The drawing under review shows one solid part. Ordinate dimensions are in mm from its lowest x, y, z. A direction names the side the tool comes from. Round coordinates to 2 decimals unless told otherwise and drop trailing zeros. Write each loop counter-clockwise with the first axis right and the second up, starting at its lowest first coordinate (ties: lowest second). Pieces come first, ordered by that corner, then holes. Notation, with made-up numbers: (30.5, 15.5) -> (55.5, 15.5) arc R13 ccw to (55.5, 28.5) -> close; hole circle Ø6 at (2, -3). An arc over 180 degrees is marked (long way). Answer in a Markdown table with one row per item.
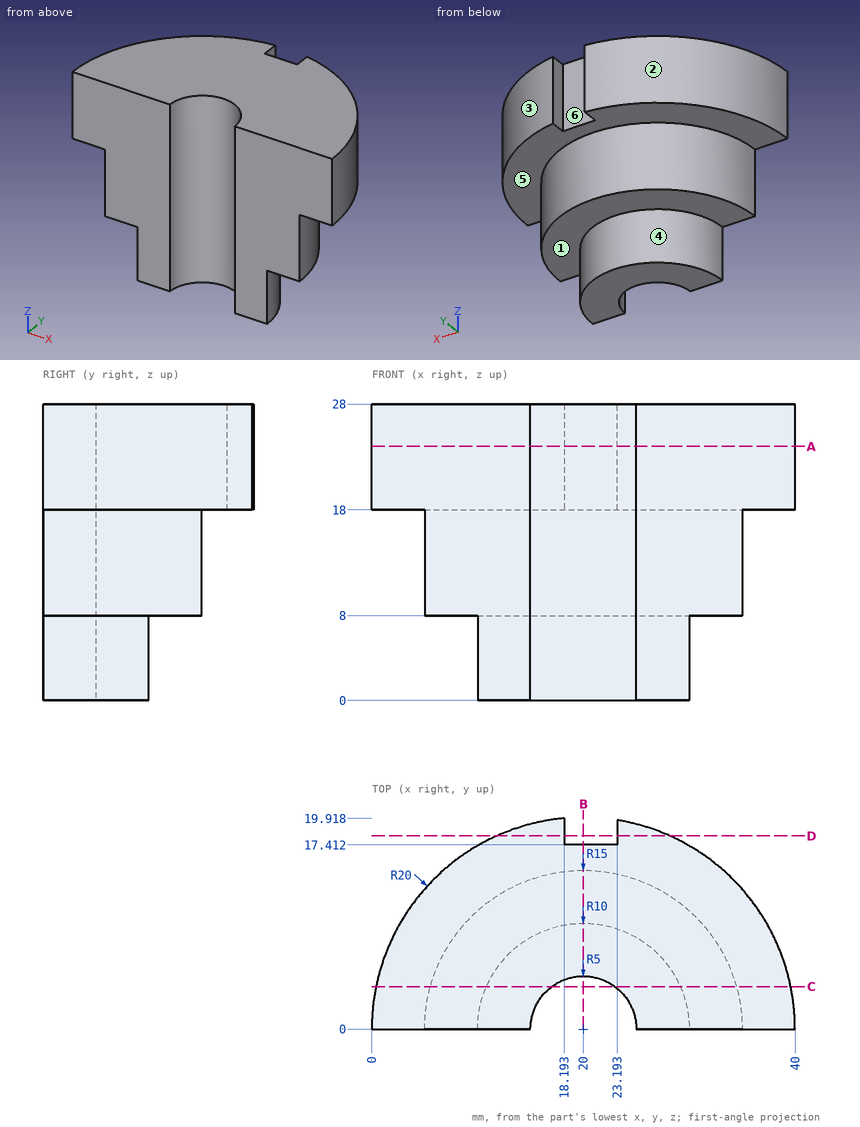
1) Mouldability with a two-part tool opening along X and no side actions: class the marked faces 3, 4, 5 and 6 as pulls with the +X half, pulls with the -X half, needs draft (parallel to the pull), parting line crosses it, or undercut.
Solved:
| item | result |
|---|---|
| face 3 | pulls with the +X half |
| face 4 | parting line crosses it |
| face 5 | needs draft |
| face 6 | undercut |
2) Consider section C-C on y = 4. State the section outline as (x, z) points (1 decimal).
Solved:
| item | result |
|---|---|
| outline | (0.4, 18) -> (5.5, 18) -> (5.5, 8) -> (10.8, 8) -> (10.8, 0) -> (17, 0) -> (17, 28) -> (0.4, 28) -> close; (23, 0) -> (29.2, 0) -> (29.2, 8) -> (34.5, 8) -> (34.5, 18) -> (39.6, 18) -> (39.6, 28) -> (23, 28) -> close |
3) Consider section D-D on y = 18.25. State the section outline as (x, z) points, then the cut area to 3 significant figures.
Solved:
| item | result |
|---|---|
| outline | (11.82, 18) -> (18.19, 18) -> (18.19, 28) -> (11.82, 28) -> close; (23.19, 18) -> (28.18, 18) -> (28.18, 28) -> (23.19, 28) -> close |
| area | 114 mm² |
4) For the marked faces 1 and 2, list the 3-axis set-ups (+Z, -Z, +X, -X, +Y, -Y) from which the entire face can be reached by the end or side of a thin tool; tool diameter is ignored.
Solved:
| item | result |
|---|---|
| face 1 | -Z, +Y |
| face 2 | +Z, -Z, -X, +Y |
5) Clearance check with flat-ended pins moving along their axes: pin 1 Ø2.5 at (x, z) = (20.5, 24.5) entering from +Y; pin 2 Ø1.5 at (x, y) = (13, 13.5) entering from -Z; pin 3 Ø2 at (y, z) = (4, 16.5) entering from -X. State where each tip first meets the part, or that it passes through.
Solved:
| item | result |
|---|---|
| pin 1 | y = 17.41 |
| pin 2 | z = 8 |
| pin 3 | x = 5.3 |
6) For line 1 (Z direction, x = 6.5, y = 13.25); line 2 (Z direction, x = 29, y = 7); line 3 (X direction, y = 1, z = 14.5), list the stretches that pass through material, from the lowest coordinate up. Write a range as [from, to].
Solved:
| item | result |
|---|---|
| line 1 | [18, 28] |
| line 2 | [8, 28] |
| line 3 | [5.03, 15.1], [24.9, 34.97] |
7) Consider section A-A on z = 24. State the section outline as (x, y) points.
Solved:
| item | result |
|---|---|
| outline | (0, 0) -> (15, 0) arc R5 cw to (25, 0) -> (40, 0) arc R20 ccw to (23.19, 19.74) -> (23.19, 17.41) -> (18.19, 17.41) -> (18.19, 19.92) arc R20 ccw to start |
8) Consider section B-B on x = 20. State the section outline as (y, z) points, then the cut area to 3 significant figures.
Solved:
| item | result |
|---|---|
| outline | (5, 0) -> (10, 0) -> (10, 8) -> (15, 8) -> (15, 18) -> (17.41, 18) -> (17.41, 28) -> (5, 28) -> close |
| area | 264 mm² |
